Study the drawing (mm; zero at the part's minimum x, y, z) and answer. A direction names the side the tool comes from. Coordinates: 2 decimals unless noted, no trailing zeros. Loops run counter-clockwise (first coordinate to the right, second up) from the corner with the lowest first, then second, coordinate; pieces in that order, holes last.
Q1. Flat-ended cylindrical pins translate along their axes: P1, Ø3, axis at y = 5, z = 5, coming from the +X side; P2, Ø2.5, axis at y = 4, z = 3.5, coming from the -X side; P3, Ø3, axis at x = 4.5, z = 4.5, coming from the +Y side. Find the tip coordinate at first contact, or state that the pin passes through.
Q2. The mould has two halves that part along Y. Classify the marked faces 3, 4 and 5: pulls with the +Y half, pulls with the -Y half, needs draft (parallel to the pull), parting line crosses it, or undercut.
Q3. Section B-B (y = 5) is taken. Give the vertices of the cut face in (x, z).
Q4. Which of the six approach directions +Z, -Z, +X, -X, +Y, -Y give full straight-line access (tool end or side, diameter ignored) to the marked faces 1 and 2?
Q5. Section D-D (z = 1.75) is taken. Give the vertices of the cut face in (x, y).
Q6. A straight line is drawn through the part: line 1 (Z direction, x = 5, y = 0.45). Find the intervals that lie inside material, in ascending order.
Q7. Section A-A (z = 5) is taken. Give the vertices of the cut face in (x, y).
Q8. Section C-C (x = 5) is taken. Give the vertices of the cut face in (y, z).
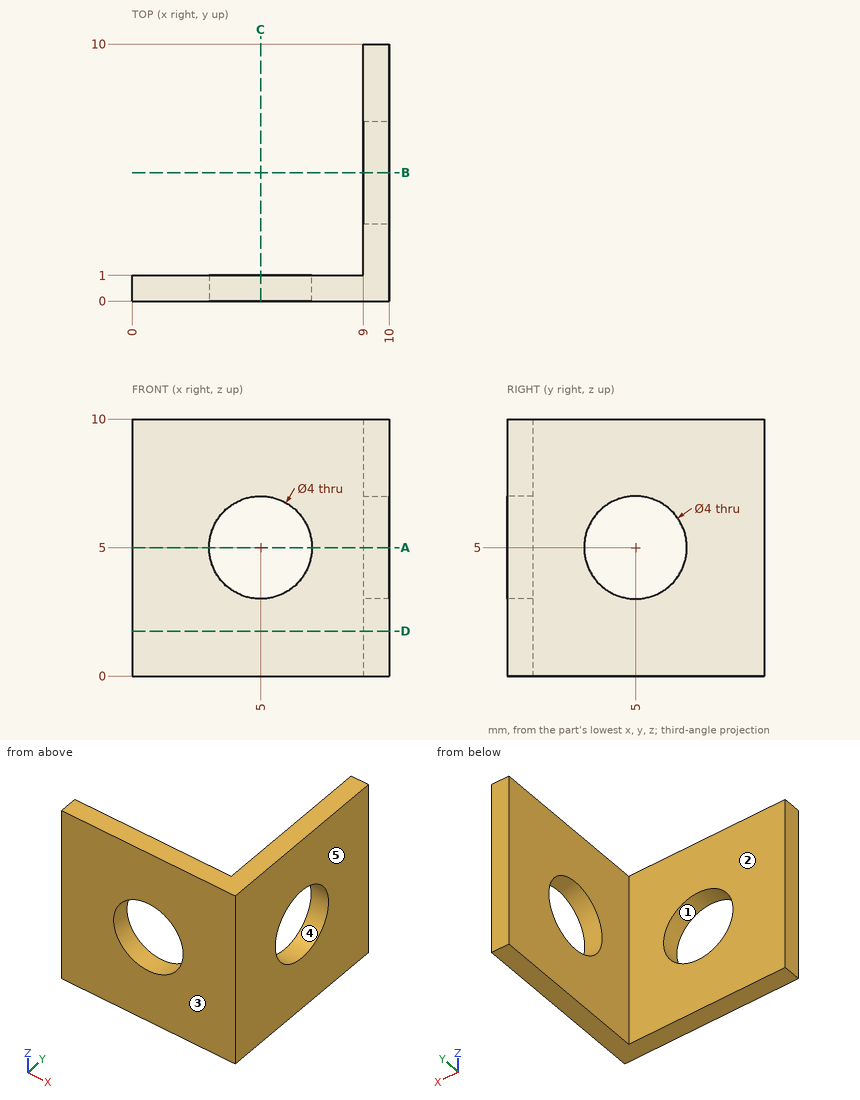
Numbers:
1. P1: passes through
1. P2: stops at x = 9
1. P3: stops at y = 1
2. face 3: pulls with the -Y half
2. face 4: undercut
2. face 5: needs draft
3. outline: (9, 0) - (10, 0) - (10, 3) - (9, 3) - close; (9, 7) - (10, 7) - (10, 10) - (9, 10) - close
4. face 1: +Y, -Y
4. face 2: +Z, -Z, -X, +Y
5. outline: (0, 0) - (10, 0) - (10, 10) - (9, 10) - (9, 1) - (0, 1) - close
6. line 1: z = 0 to 3, 7 to 10
7. outline: (0, 0) - (3, 0) - (3, 1) - (0, 1) - close; (7, 0) - (10, 0) - (10, 3) - (9, 3) - (9, 1) - (7, 1) - close; (9, 7) - (10, 7) - (10, 10) - (9, 10) - close
8. outline: (0, 0) - (1, 0) - (1, 3) - (0, 3) - close; (0, 7) - (1, 7) - (1, 10) - (0, 10) - close
